Autodesk Inventor part; units mm, degrees
ref_plane "Mid Plane" through (152.4, 0, 0) normal (1, 0, 0) x (0, 0, -1)
ref_plane "Horizontal Midplane" through (-25.4, 0, 0) normal (0, 1, 0) x (1, 0, 0)
ref_plane "YZ Plane" through (0, 0, 0) normal (1, 0, 0) x (0, 1, 0)
sketch "Sketch1" plane through (0, 0, 0) normal (1, 0, 0) x (0, 1, 0)
  circle A0 centre (0, 0) radius 3.7474
extrude "Black Shaft" add sketch "Sketch1" along normal blind 304.8
sketch "Sketch3" plane through (304.8, 0, 0) normal (1, 0, 0) x (0, 0, -1)
  circle A0 centre (0, 0) radius 2.3813
  dimension "d2" = 4.7625
extrude "Screwed Shaft" add sketch "Sketch3" along normal blind 12.7 and the other way blind 317.5
ref_plane "Mid Plane" through (152.4, 0, 0) normal (1, 0, 0) x (0, 0, -1)
sketch "Sketch4" plane through (0, 0, 0) normal (0, 1, 0) x (-1, 0, 0)
  circle A0 centre (25.4, 0) radius 13.0969
  line L0 (12.7, -2.3813) -> (12.7, 2.3813) construction
  circle A1 centre (25.4, 0) radius 9.525
  point P0 (0, 0)
  dimension "d7" = 26.1938
  dimension "d8" = 12.7
  dimension "d9" = 19.05
extrude "Rod End1" add sketch "Sketch4" along normal mid plane 4.7625
mirror "Rod End2" about plane through (152.4, 0, 0) normal (1, 0, 0) of "Rod End1"
ref_plane "Horizontal Midplane" through (-25.4, 0, 0) normal (0, 1, 0) x (1, 0, 0)
properties part number "Tie Rods" material "Aluminum 6061"
Input: part model. Units: mm. Frame: model coordinates. A direction names the side the tool comes from. Coordinates: 2 decimals unless noted, no trailing zeros. Loops run counter-clockwise (first coordinate to the right, second up) from the corner with the lowest first, then second, coordinate; pieces in that order, holes last.
Q1. Line query: line 1 along Z through (x, y) = (-25.4, -0.8) (3 decimals); line 2 along X through (y, z) = (2, -5.5); line 3 along Z through (x, y) = (212, 0). Output: solid intervals per line, ascending.
Results are:
line 1: z = -13.097 to -9.525, 9.525 to 13.097
line 2: x = -37.29 to -33.18, -17.62 to -13.51, 318.31 to 322.42, 337.98 to 342.09
line 3: z = -3.75 to 3.75
Q2. Section A-A, the plane y = 0. Return the cut outline in (x, z) (3 decimals), and give its area (3 significant figures).
Results are:
outline: (-12.521, -2.381) - (0, -2.381) - (0, -3.747) - (304.8, -3.747) - (304.8, -2.381) - (317.321, -2.381) arc R13.097 ccw (long way) to (317.321, 2.381) - (304.8, 2.381) - (304.8, 3.747) - (0, 3.747) - (0, 2.381) - (-12.521, 2.381) arc R13.097 ccw (long way) to start; hole circle Ø19.05 at (-25.4, 0); hole circle Ø19.05 at (330.2, 0)
area: 2,910 mm2
Q3. Section B-B, the plane x = -25.4. Return the cut outline in (y, z) (3 decimals), and give its area (3 significant figures).
Results are:
outline: (-2.381, -13.097) - (2.381, -13.097) - (2.381, -9.525) - (-2.381, -9.525) - close; (-2.381, 9.525) - (2.381, 9.525) - (2.381, 13.097) - (-2.381, 13.097) - close
area: 34.0 mm2
Q4. Set-up query: faces 4 (the flat face through (-26, -2.381, -10)), 5 (the flat face through (304.8, 2.45, -0.78)), 6 (the flat face through (329, 2.381, -10)), 7 (the flat face through (-26, 2.381, -10)). Return all of +Z, -Z, +X, -X, +Y, -Y with unobstructed straight access to the full face (end or side cutting, diameter ignored); none if empty.
Results are:
face 4: +Z, -Z, -X, -Y
face 5: none
face 6: +Z, -Z, +X, +Y
face 7: +Z, -Z, -X, +Y
Q5. Mould query, pull axis X, two halves, no side actions, for faces 1 (the flat face through (329, -2.381, -10)), 2 (the cylindrical face through (-15.884, 0.033, 0.419)), 3 (the cylindrical face through (320.684, 0.033, -0.419)). Classes: +X half, -X half, draft (parallel to the pull), parting line (faces both ways), or undercut.
Results are:
face 1: draft
face 2: undercut
face 3: undercut
Q6. Contact query for flat-ended pins moving along their axis: pin 1 (2 mm diameter, centred on y = -1, z = 1.5, fed in from +X); pin 2 (1 mm diameter, centred on x = 268.5, y = -2, fed in from +Z); pin 3 (1.5 mm diameter, centred on x = 26.5, y = 0.5, fed in from +Z). Output: stop coordinate, or through.
Results are:
pin 1: stops at x = 343.29
pin 2: stops at z = 3.43
pin 3: stops at z = 3.75
